from build123d import *

# Parameters (mm, degrees)
SKETCH_W     = 50
SKETCH_H     = 14
PAD_DEPTH    = 3
SKETCH001_W  = 14
SKETCH001_H  = 2
PAD001_DEPTH = 39
POCKET_DEPTH = 2
FILLET_R     = 4


with BuildPart() as part:
    # Sketch → Pad (new body)
    with BuildSketch(Plane.XY):
        with Locations((25, 7)):
            Rectangle(SKETCH_W, SKETCH_H)
    extrude(amount=PAD_DEPTH)

    # Sketch001 (on Face6 of Pad) → Pad001 (join)
    with BuildSketch(Plane.XY.offset(3)):
        with Locations((25, 13)):
            Rectangle(SKETCH001_W, SKETCH001_H)
    extrude(amount=PAD001_DEPTH)

    # Sketch002 (on Face8 of Pad001) → Pocket (cut)
    with BuildSketch(Plane.XZ.offset(-12)):
        with BuildLine():
            ThreePointArc((26.55, 39), (25, 40.55), (23.45, 39))
            Line((23.45, 39), (23.45, 6))
            ThreePointArc((23.45, 6), (25, 4.45), (26.55, 6))
            Line((26.55, 39), (26.55, 6))
        make_face()
    extrude(amount=-POCKET_DEPTH, mode=Mode.SUBTRACT)

    # Fillet
    fillet_edges = [part.edges().sort_by_distance(p)[0] for p in [
        (0, 0, 1.5),
        (50, 0, 1.5),
        (18, 13, 42),
        (32, 13, 42),
        (0, 14, 1.5),
        (50, 14, 1.5),
    ]]
    fillet(fillet_edges, radius=FILLET_R)


solid = part.part
Check sheet for the modelled part. Datum: model origin and axes. Units: mm. A direction names the side the tool comes from. Give positions to 0.01 mm unless a question says otherwise; leave off trailing zeros. Loops run counter-clockwise (first coordinate to the right, second up) from the corner with the lowest first, then second, coordinate; pieces in that order, holes last. Notation, with made-up numbers: M 26.25,64.5 L 39.25,64.5 A22 cw 39.25,85.5 Z; hole C -4.75,-31.75 d9. An arc over 180 degrees is marked long. Answer as a JSON object with one key per item and string values. Group by question number.
Q1. Access from +Z, -Z, +X, -X, +Y, -Y to the whole of each face (thin tool, end or side, straight path). Record for faces 1 (the flat face through (32, 13, 20)), 2 (the flat face through (23, 12, 22)), 3 (the flat face through (26.55, 13, 23)).
Q2. Cross-section at C-C on y = 13.25. Record the cut outline in (x, z).
Q3. Go/stop test with flat-tipped pins: P1, Ø4, axis at x = 39.5, y = 6.5, coming from the +Z side; P2, Ø0.6, axis at y = 13.5, z = 23, coming from the -X side; P3, Ø1.6, axis at y = 13, z = 12.5, coming from the +X side. Record where each tip stops, or that it passes through.
Q4. Material ranges on line 1 along X through (y, z) = (13.25, 19.5); line 2 along Z through (x, y) = (11.5, 9.25); line 3 along Y through (x, z) = (29, 9), recorded low to high. Write a range as [from, to].
Q5. Cross-section at D-D on x = 13.5. Record the cut outline in (y, z), then the cut area to 3 significant figures.
Q6. Release check for a two-part mould opening along X. For faces 4 (the flat face through (18, 13, 20)), 5 (the flat face through (25, 7, 3)), 6 (the flat face through (23.45, 13, 23)) record: released by +X, released by -X, zero draft, split by the parting line, or undercut.
Q7. Cross-section at B-B on x = 25. Record the cut outline in (y, z), then the cut area to 3 significant figures.
Q8. Cross-section at A-A on z = 18.5. Record the cut outline in (x, y).
Evaluation:
{
 "1": {"face 1": "+Z, +X, +Y, -Y", "face 2": "+Z, +X, -X, -Y", "face 3": "+Y, -Y"},
 "2": {"outline": "M 1.67,0 L 48.33,0 L 48.33,3 L 32,3 L 32,38 A4 ccw 28,42 L 22,42 A4 ccw 18,38 L 18,3 L 1.67,3 Z; hole M 23.45,6 A1.55 ccw 26.55,6 L 26.55,39 A1.55 ccw 23.45,39 Z"},
 "3": {"P1": "stops at z = 3", "P2": "stops at x = 18", "P3": "stops at x = 32"},
 "4": {"line 1": "x = [18, 23.45], [26.55, 32]", "line 2": "z = [0, 3]", "line 3": "y = [12, 14]"},
 "5": {"outline": "M 0,0 L 14,0 L 14,3 L 0,3 Z", "area": "42.0 mm2"},
 "6": {"face 4": "released by -X", "face 5": "zero draft", "face 6": "undercut"},
 "7": {"outline": "M 0,0 L 14,0 L 14,4.45 L 12,4.45 L 12,3 L 0,3 Z; M 12,40.55 L 14,40.55 L 14,42 L 12,42 Z", "area": "47.8 mm2"},
 "8": {"outline": "M 18,12 L 23.45,12 L 23.45,14 L 18,14 Z; M 26.55,12 L 32,12 L 32,14 L 26.55,14 Z"}
}
